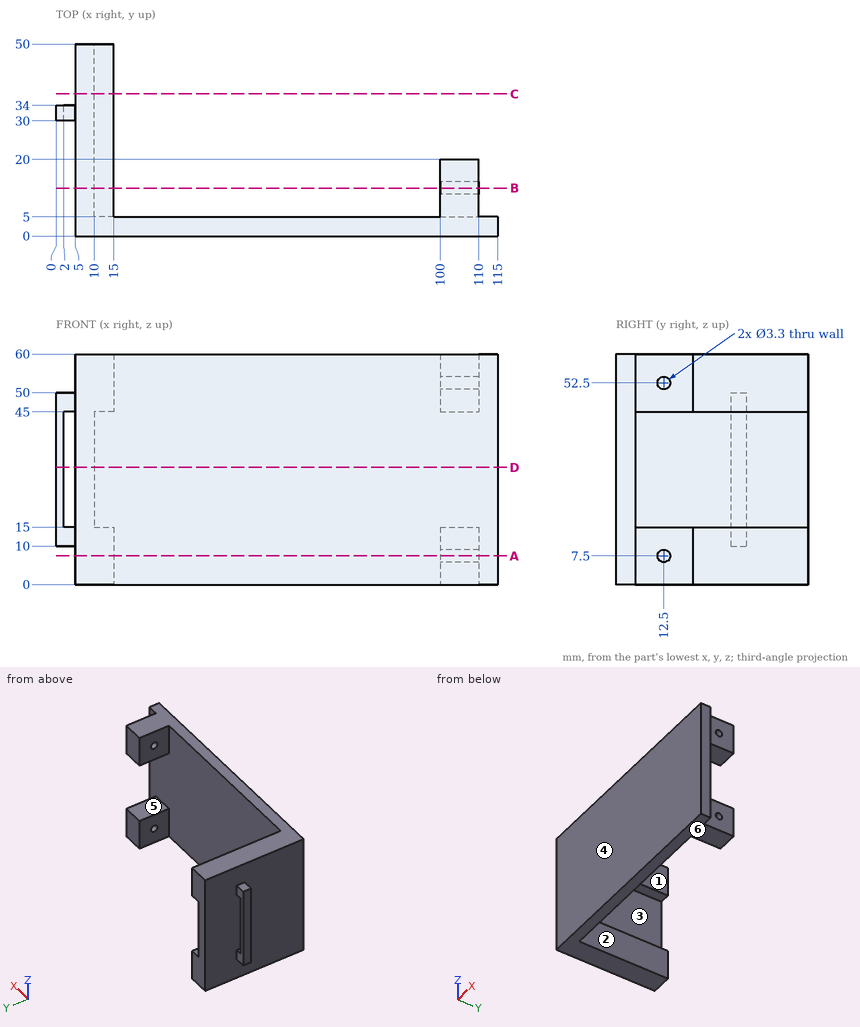
Verification items for this drawing (mm, ordinates from the low corner). A direction names the side the tool comes from. Round coordinates to 2 decimals unless told otherwise and drop trailing zeros. Loops run counter-clockwise (first coordinate to the right, second up) from the corner with the lowest first, then second, coordinate; pieces in that order, holes last. Notation, with made-up numbers: (58, 81.25) - (99, 81.25) arc R15 ccw to (99, 92.25) - close; hole circle Ø2 at (14, 67). An arc over 180 degrees is marked (long way). Answer as CSV lines item,"result". Start each with the question number.
Item 1: Section check B-B (y = 12.5). Record the boundary of the cut face in (x, z), and give its area (3 significant figures).
Item 2: Section check A-A (z = 7.5). Record the boundary of the cut face in (x, y), and give its area (3 significant figures).
Item 3: Release check for a two-part mould opening along X. For the marked faces 1, 2, 3 and 4 record: +X half, -X half, draft (parallel to the pull), parting line (faces both ways), or undercut.
Item 4: Scan lines: line 1 (Z direction, x = 10.5, y = 24); line 2 (Z direction, x = 105, y = 12); line 3 (Y direction, x = 106.25, z = 7.5). Record each from-to range of solid material in increasing order. Write a range as [from, to].
Item 5: Section check D-D (z = 30.5). Record the boundary of the cut face in (x, y).
Item 6: Section check C-C (y = 37). Record the boundary of the cut face in (x, z), and give its area (3 significant figures).
Item 7: Depth check by flat-ended pin: P1, Ø10, axis at y = 40.5, z = 42.5, coming from the -X side; P2, Ø1.2, axis at x = 1.5, y = 33, coming from the -Z side; P3, Ø5.5, axis at x = 1.5, z = 32.5, coming from the +Y side. Enter the tip coordinate at first touch or a pass-through.
Item 8: Set-up check for the marked faces 5 and 6: record each of +Z, -Z, +X, -X, +Y, -Y from which the full face is reachable in a straight line by a thin tool's end or side.
Report:
1,outline,"(5, 0) - (15, 0) - (15, 15) - (10, 15) - (10, 45) - (15, 45) - (15, 60) - (5, 60) - close; (100, 0) - (110, 0) - (110, 5.85) - (100, 5.85) - close; (100, 9.15) - (110, 9.15) - (110, 15) - (100, 15) - close; (100, 45) - (110, 45) - (110, 50.85) - (100, 50.85) - close; (100, 54.15) - (110, 54.15) - (110, 60) - (100, 60) - close"
1,area,"684 mm2"
2,outline,"(5, 0) - (115, 0) - (115, 5) - (110, 5) - (110, 10.85) - (100, 10.85) - (100, 5) - (15, 5) - (15, 50) - (5, 50) - close; (100, 14.15) - (110, 14.15) - (110, 20) - (100, 20) - close"
2,area,"1,120 mm2"
3,face 1,"undercut"
3,face 2,"undercut"
3,face 3,"+X half"
3,face 4,"draft"
4,line 1,"z = [0, 15], [45, 60]"
4,line 2,"z = [0, 5.93], [9.07, 15], [45, 50.93], [54.07, 60]"
4,line 3,"y = [0, 10.85], [14.15, 20]"
5,outline,"(0, 30) - (2, 30) - (2, 34) - (0, 34) - close; (5, 0) - (115, 0) - (115, 5) - (10, 5) - (10, 50) - (5, 50) - close"
6,outline,"(5, 0) - (15, 0) - (15, 15) - (10, 15) - (10, 45) - (15, 45) - (15, 60) - (5, 60) - close"
6,area,"450 mm2"
7,P1,"stops at x = 5"
7,P2,"stops at z = 10"
7,P3,"stops at y = 34"
8,face 5,"+X, +Y"
8,face 6,"-Z, +X, -X, +Y, -Y"
